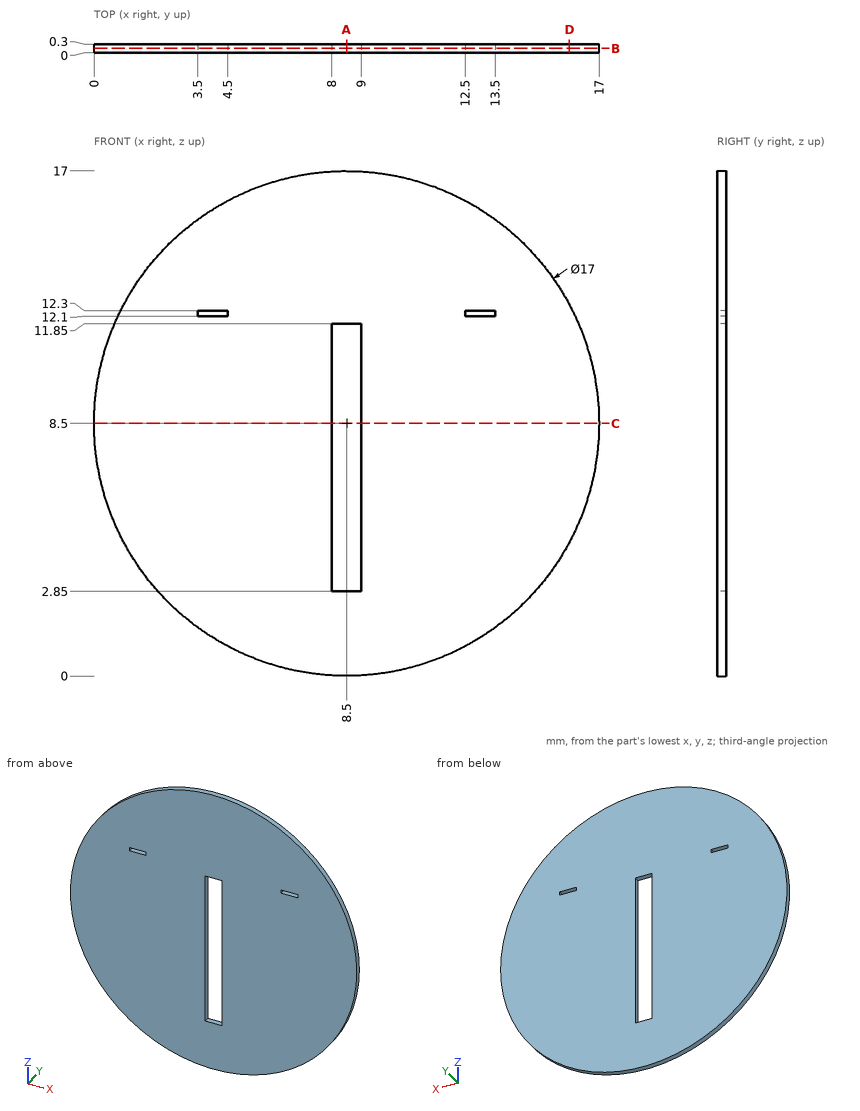
Source: three-view drawing plus pictorial views. Frame: mm from the lowest corner of the part. Round coordinates to 2 decimals unless told otherwise and drop trailing zeros. Order: outer loops, then holes, each group sorted by start corner. A loop starts at its lowest first (then second) coordinate and runs counter-clockwise, first axis right, second up. Notation, with made-up numbers: (-15.5, 13) -> (19.5, 13) arc R16 cw to (19.5, 42) -> close; hole circle Ø4 at (5, 76). An arc over 180 degrees is marked (long way). Use one line per item in the form item = value.
(1) Section B-B on y = 0.15. Return loops of the section in (x, z), and give its area (3 significant figures).
Results list:
outline = circle Ø17 at (8.5, 8.5); hole (3.5, 12.1) -> (4.5, 12.1) -> (4.5, 12.3) -> (3.5, 12.3) -> close; hole (8, 2.85) -> (9, 2.85) -> (9, 11.85) -> (8, 11.85) -> close; hole (12.5, 12.1) -> (13.5, 12.1) -> (13.5, 12.3) -> (12.5, 12.3) -> close
area = 218 mm^2
(2) Ray query, probe 1 along Z at (x, y) = (8.5, 0.15); probe 2 along X at (y, z) = (0.1, 4.5); probe 3 along Z at (x, y) = (13, 0.25). Return the intervals inside material, ascending. Write a range as [from, to].
Results list:
probe_1 = [0, 2.85], [11.85, 17]
probe_2 = [1, 8], [9, 16]
probe_3 = [1.29, 12.1], [12.3, 15.71]
(3) Section D-D on x = 16. Return loops of the section in (y, z), and give its area (3 significant figures).
Results list:
outline = (0, 4.5) -> (0.3, 4.5) -> (0.3, 12.5) -> (0, 12.5) -> close
area = 2.40 mm^2
(4) Section C-C on z = 8.5. Return loops of the section in (x, y), and give its area (3 significant figures).
Results list:
outline = (0, 0) -> (8, 0) -> (8, 0.3) -> (0, 0.3) -> close; (9, 0) -> (17, 0) -> (17, 0.3) -> (9, 0.3) -> close
area = 4.80 mm^2
(5) Section A-A on x = 8.5. Return loops of the section in (y, z), and give its area (3 significant figures).
Results list:
outline = (0, 0) -> (0.3, 0) -> (0.3, 2.85) -> (0, 2.85) -> close; (0, 11.85) -> (0.3, 11.85) -> (0.3, 17) -> (0, 17) -> close
area = 2.40 mm^2
